Build history of the part. All positions in model axes, mm. A direction names the side the tool comes from. Coordinates: 2 decimals unless noted, no trailing zeros. Loops run counter-clockwise (first coordinate to the right, second up) from the corner with the lowest first, then second, coordinate; pieces in that order, holes last. Notation, with made-up numbers: (-19, 0.5) - (34, 0.5) arc R16 cw to (34, 14.5) - close; hole circle Ø1 at (9.5, 45.25). An arc over 180 degrees is marked (long way). One line per item, written item: value.
Autodesk Inventor part; units mm, degrees
ref_plane "Work Plane1" through (0, 0, 0) normal (0, 0, 1) x (1, 0, 0)
ref_plane "Work Plane3" through (204.5669, 33.2743, 819.985) normal (0, 0, 1) x (1, 0, 0)
ref_plane "Work Plane4" through (204.5669, 0, 909.6375) normal (0, 0, 1) x (1, 0, 0)
ref_plane "Work Plane1" through (0, 0, 0) normal (0, 0, 1) x (1, 0, 0)
ref_plane "Work Plane3" through (204.5669, 33.2743, 819.985) normal (0, 0, 1) x (1, 0, 0)
ref_plane "Work Plane4" through (204.5669, 0, 909.6375) normal (0, 0, 1) x (1, 0, 0)
sketch "Sketch1" plane through (0, 0, 0) normal (0, 0, 1) x (1, 0, 0)
  arc A0 (-113.2188, 0) -> (-109.7581, 3.4607) centre (-113.2188, 3.4607) ccw
  line L0 (-109.7581, 17.1767) -> (-109.7581, 3.4607)
  arc A1 (-109.7581, 17.1767) -> (-114.8063, 22.225) centre (-114.8063, 17.1767) ccw
  line L1 (-115.8223, 22.225) -> (-114.8063, 22.225)
  arc A2 (-115.8223, 22.225) -> (-119.2831, 18.7642) centre (-115.8223, 18.7642) ccw
  line L2 (-119.2831, 16.4211) -> (-119.2831, 18.7642)
  arc A3 (-119.2831, 16.4211) -> (-116.6161, 16.4211) centre (-117.9496, 16.4211) ccw
  line L3 (-116.6161, 18.7642) -> (-116.6161, 16.4211)
  arc A4 (-115.8223, 19.558) -> (-116.6161, 18.7642) centre (-115.8223, 18.7642) ccw
  line L4 (-114.8063, 19.558) -> (-115.8223, 19.558)
  arc A5 (-112.4251, 17.1767) -> (-114.8063, 19.558) centre (-114.8063, 17.1767) ccw
  line L5 (-112.4251, 3.4607) -> (-112.4251, 17.1767)
  arc A6 (-113.2188, 2.667) -> (-112.4251, 3.4607) centre (-113.2188, 3.4607) ccw
  line L6 (-147.5723, 2.667) -> (-113.2188, 2.667)
  arc A7 (-148.3661, 3.4607) -> (-147.5723, 2.667) centre (-147.5723, 3.4607) ccw
  line L7 (-148.3661, 17.1767) -> (-148.3661, 3.4607)
  arc A8 (-145.9848, 19.558) -> (-148.3661, 17.1767) centre (-145.9848, 17.1767) ccw
  line L8 (-144.9688, 19.558) -> (-145.9848, 19.558)
  arc A9 (-144.1751, 18.7642) -> (-144.9688, 19.558) centre (-144.9688, 18.7642) ccw
  line L9 (-144.1751, 16.4211) -> (-144.1751, 18.7642)
  arc A10 (-144.1751, 16.4211) -> (-141.5081, 16.4211) centre (-142.8416, 16.4211) ccw
  line L10 (-141.5081, 18.7642) -> (-141.5081, 16.4211)
  arc A11 (-141.5081, 18.7642) -> (-144.9688, 22.225) centre (-144.9688, 18.7642) ccw
  line L11 (-145.9848, 22.225) -> (-144.9688, 22.225)
  arc A12 (-145.9848, 22.225) -> (-151.0331, 17.1767) centre (-145.9848, 17.1767) ccw
  line L12 (-151.0331, 3.4607) -> (-151.0331, 17.1767)
  arc A13 (-151.0331, 3.4607) -> (-147.5723, 0) centre (-147.5723, 3.4607) ccw
  line L13 (-113.2188, 0) -> (-147.5723, 0)
  point P0 (0, 0)
extrude "Extrusion1" add sketch "Sketch1" along normal up to surface (909.6375 mm away)
properties part number "Horizontal-Unistrut-Tower-Connector-19-25"
Item 1: Pull direction X, two halves, no side cores. Call faces 3 (the face through (-112.425, 10, 448)), 4 (the face through (-130, 2, 0)), 5 (the face through (-151.033, 10, 448)): released by +X, released by -X, zero draft, split by the parting line, or undercut.
Check result:
face 3: undercut
face 4: zero draft
face 5: released by -X
Item 2: Tool access for faces 1 (the face through (-130, 2, 909.638)), 2 (the face through (-148.366, 10, 448)): list every direction of +Z, -Z, +X, -X, +Y, -Y with a clear straight run to the whole face (end or side of a thin tool).
Check result:
face 1: +Z, +X, -X, +Y, -Y
face 2: +Z, -Z
Item 3: Probe probe 1 along X at (y, z) = (18, 576); probe 2 along X at (y, z) = (10, 181); probe 3 along Y at (x, z) = (-116, 121.5). List the from-to ranges inside material, lowest first. Write a range as from..to.
Check result:
probe 1: x = -150.97..-148.22, -144.18..-141.51, -119.28..-116.62, -112.57..-109.83
probe 2: x = -151.03..-148.37, -112.43..-109.76
probe 3: y = 0..2.67, 19.54..22.22
Item 4: Cut at C-C, the plane x = -134.5. Write the cut outline in (y, z), then the cut area to 3 significant figures.
Check result:
outline: (0, 0) - (2.67, 0) - (2.67, 909.64) - (0, 909.64) - close
area: 2,430 mm^2
Item 5: Cut at B-B, the plane z = 76. Write the cut outline in (x, y) (1 decimal), then the cut area to 3 significant figures.
Check result:
outline: (-151, 3.5) arc R3.5 ccw to (-147.6, 0) - (-113.2, 0) arc R3.5 ccw to (-109.8, 3.5) - (-109.8, 17.2) arc R5 ccw to (-114.8, 22.2) - (-115.8, 22.2) arc R3.5 ccw to (-119.3, 18.8) - (-119.3, 16.4) arc R1.3 ccw to (-116.6, 16.4) - (-116.6, 18.8) arc R0.8 cw to (-115.8, 19.6) - (-114.8, 19.6) arc R2.4 cw to (-112.4, 17.2) - (-112.4, 3.5) arc R0.8 cw to (-113.2, 2.7) - (-147.6, 2.7) arc R0.8 cw to (-148.4, 3.5) - (-148.4, 17.2) arc R2.4 cw to (-146, 19.6) - (-145, 19.6) arc R0.8 cw to (-144.2, 18.8) - (-144.2, 16.4) arc R1.3 ccw to (-141.5, 16.4) - (-141.5, 18.8) arc R3.5 ccw to (-145, 22.2) - (-146, 22.2) arc R5 ccw to (-151, 17.2) - close
area: 255 mm^2
Item 6: Cut at A-A, the plane y = 9. Write the cut outline in (x, z), then the cut area to 3 significant figures.
Check result:
outline: (-151.03, 0) - (-148.37, 0) - (-148.37, 909.64) - (-151.03, 909.64) - close; (-112.43, 0) - (-109.76, 0) - (-109.76, 909.64) - (-112.43, 909.64) - close
area: 4,850 mm^2
